```python
from build123d import *

# Parameters (mm, degrees)
SKETCH1_R           = 5.5
BOSS_EXTRUDE1_DEPTH = 6.3
SKETCH2_R           = 4.915
BOSS_EXTRUDE2_DEPTH = 8
SKETCH3_R           = 7.5
BOSS_EXTRUDE3_DEPTH = 3.2
SKETCH5_R           = 2
CUT_EXTRUDE1_DEPTH  = 21.46338193


with BuildPart() as part:
    # Sketch1 → Boss-Extrude1 (new body)
    with BuildSketch(Plane(origin=(0, 0, 0), x_dir=(0, 0, -1), z_dir=(1, 0, 0))):
        Circle(SKETCH1_R)
    extrude(amount=BOSS_EXTRUDE1_DEPTH)

    # Sketch2 → Boss-Extrude2 (add)
    with BuildSketch(Plane(origin=(6.3, 0, 0), x_dir=(0, 0, -1), z_dir=(1, 0, 0))):
        Circle(SKETCH2_R)
    extrude(amount=BOSS_EXTRUDE2_DEPTH)

    # Sketch3 → Boss-Extrude3 (add)
    with BuildSketch(Plane(origin=(14.3, 0, 0), x_dir=(0, 0, -1), z_dir=(1, 0, 0))):
        Circle(SKETCH3_R)
    extrude(amount=BOSS_EXTRUDE3_DEPTH)

    # Sketch5 → Cut-Extrude1 (cut, through all)
    with BuildSketch(Plane.ZY):
        Circle(SKETCH5_R)
    extrude(amount=-CUT_EXTRUDE1_DEPTH, mode=Mode.SUBTRACT)


solid = part.part
```
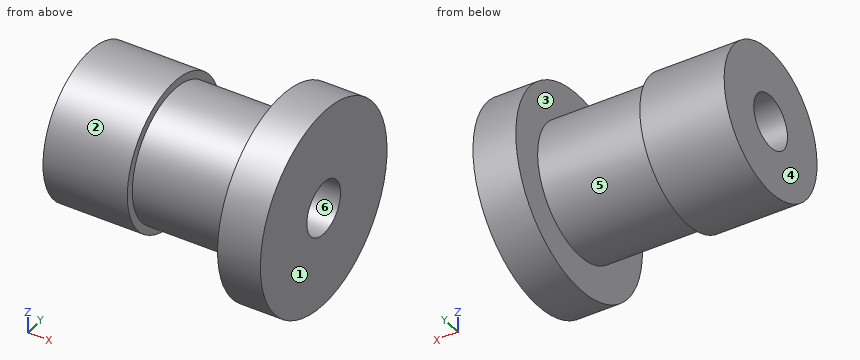
Design review of the part built by this model. Coordinates are the model's own, in mm. Face numbers are marked on the shaded views. A direction names the side the tool comes from. Coordinates: 2 decimals unless noted, no trailing zeros. Loops run counter-clockwise (first coordinate to the right, second up) from the corner with the lowest first, then second, coordinate; pieces in that order, holes last.
Q1. We need section D-D on z = -4. State the section outline as (x, y) points.
Reported:
outline: (0, -3.77) - (6.3, -3.77) - (6.3, -2.86) - (14.3, -2.86) - (14.3, -6.34) - (17.5, -6.34) - (17.5, 6.34) - (14.3, 6.34) - (14.3, 2.86) - (6.3, 2.86) - (6.3, 3.77) - (0, 3.77) - close
Q2. We need section C-C on x = 3.5. State the section outline as (y, z) points, and give its area (3 significant figures).
Reported:
outline: circle Ø11 at (0, 0); hole circle Ø4 at (0, 0)
area: 82.5 mm2
Q3. Tool access review of the marked faces 1, 2 and 3: name each direction out of +Z, -Z, +X, -X, +Y, -Y from which nothing blocks a thin tool from reaching the whole face with its end or side.
Reported:
face 1: +Z, -Z, +X, +Y, -Y
face 2: -X
face 3: none
Q4. We need section A-A on z = 0. State the section outline as (x, y) points (3 decimals), and give its area (3 significant figures).
Reported:
outline: (0, -5.5) - (6.3, -5.5) - (6.3, -4.915) - (14.3, -4.915) - (14.3, -7.5) - (17.5, -7.5) - (17.5, -2) - (0, -2) - close; (0, 2) - (17.5, 2) - (17.5, 7.5) - (14.3, 7.5) - (14.3, 4.915) - (6.3, 4.915) - (6.3, 5.5) - (0, 5.5) - close
area: 126 mm2
Q5. To check wall thickness, follow line 1 (Y direction, x = 4.75, z = 0); line 2 (Y direction, x = 6.5, z = 0) (3 decimals); line 3 (X direction, y = 3.5, z = 3.75). State the ranges of each line that lie inside material, in increasing order.
Reported:
line 1: y = -5.5 to -2, 2 to 5.5
line 2: y = -4.915 to -2, 2 to 4.915
line 3: x = 0 to 6.3, 14.3 to 17.5
Q6. The part is to be moulded in two halves that separate along Y. For the marked faces 4, 5 and 6, say which applies: +Y half, -Y half, draft (parallel to the pull), parting line (faces both ways), or undercut.
Reported:
face 4: draft
face 5: parting line
face 6: undercut
Q7. For pin 1 (3 mm diameter, centred on y = -5, z = 5.5, fed in from -X); pin 2 (8 mm diameter, centred on x = 15, y = -5.5, fed in from -Z); pin 3 (2 mm diameter, centred on x = 8, z = -3, fed in from +Y); pin 4 (3.5 mm diameter, centred on y = 0, z = 0, fed in from -X), all flat-tipped, find the tip position at first contact; note any pin that passes through.
Reported:
pin 1: stops at x = 14.3
pin 2: stops at z = -7.35
pin 3: stops at y = 4.49
pin 4: passes through
